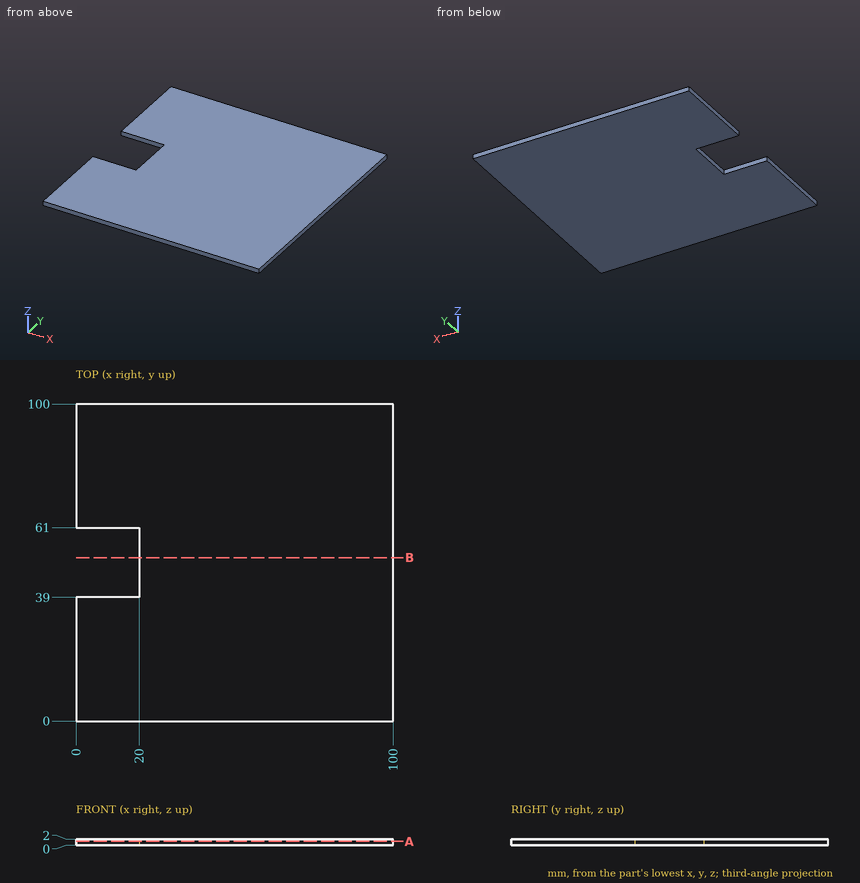
Could you check a few things on this drawing? It's one solid part, dimensions in mm from its lowest x, y, z. Coordinates: 2 decimals unless noted, no trailing zeros. Order: outer loops, then holes, each group sorted by start corner. A loop starts at its lowest first (then second) coordinate and runs counter-clockwise, first axis right, second up.
1. If we section it at A-A (z = 1.25): Please give me the cut outline in (x, y), then the cut area to 3 significant figures.
2. I'm going to push a flat-ended pin straight in: pin 1 (0.6 mm diameter, centred on y = 52.5, z = 1.5, fed in from -X). Where does the tip first touch, or does it pass through?
3. If we section it at B-B (y = 51.5): Please give me the cut outline in (x, z).
4. I need wall thicknesses on line 1 (Y direction, x = 16, z = 1.2); line 2 (X direction, y = 59, z = 1.05). Which ranges of each line are inside material? Lowest first, please.
Entries:
1. outline: (0, 0) - (100, 0) - (100, 100) - (0, 100) - (0, 61) - (20, 61) - (20, 39) - (0, 39) - close
1. area: 9,560 mm2
2. pin 1: stops at x = 20
3. outline: (20, 0) - (100, 0) - (100, 2) - (20, 2) - close
4. line 1: y = 0 to 39, 61 to 100
4. line 2: x = 20 to 100
